Geometry: final body of the model. Coordinates: model frame, mm. A direction names the side the tool comes from. Round coordinates to 2 decimals unless told otherwise and drop trailing zeros. Loops run counter-clockwise (first coordinate to the right, second up) from the corner with the lowest first, then second, coordinate; pieces in that order, holes last. Notation, with made-up numbers: M 70,-7 L 124,-7 A19 cw 124,23 Z; hole C 89,15 d2. An arc over 180 degrees is marked long. Answer as a JSON object with one key per item and string values.
from build123d import *

# Parameters (mm, degrees)
F1_DEPTH = 96.75
F2_W     = 67
F2_H     = 15
F3_DEPTH = 2.5
F4_W     = 54
F4_H     = 1
F5_DEPTH = 88
F6_W     = 45
F6_H     = 77
F7_DEPTH = 1.5
F8_R     = 1
F9_R     = 2


with BuildPart() as f1:
    # F0 (on Front) → F1 (new body)
    with BuildSketch(Plane.XZ):
        Polygon((-27.75, 0), (-27.75, -3), (-30.75, -3), (-30.75, -4.5), (30.75, -4.5), (30.75, -3), (27.75, -3), (27.75, 0), align=None)
    extrude(amount=F1_DEPTH)

    # F2 (on face) → F3 (join)
    with BuildSketch(Plane.XZ.offset(96.75)):
        with Locations((0, -8.5)):
            Rectangle(F2_W, F2_H)
    extrude(amount=F3_DEPTH)

    # F4 (on face) → F5 (cut)
    with BuildSketch(Plane(origin=(0, 0, 0), x_dir=(-1, 0, 0), z_dir=(0, 1, 0))):
        with Locations((0, -2)):
            Rectangle(F4_W, F4_H)
    extrude(amount=-F5_DEPTH, mode=Mode.SUBTRACT)

    # F6 (on face) → F7 (cut, through all)
    with BuildSketch(Plane.XY):
        with Locations((0, -42.5)):
            Rectangle(F6_W, F6_H)
    extrude(amount=-F7_DEPTH, mode=Mode.SUBTRACT)

    # F8
    f8_edges = [f1.edges().sort_by_distance(p)[0] for p in [
        (-22.5, -81, -0.75),
        (-22.5, -4, -0.75),
        (22.5, -4, -0.75),
        (22.5, -81, -0.75),
    ]]
    fillet(f8_edges, radius=F8_R)

    # F9
    f9_edges = [f1.edges().sort_by_distance(p)[0] for p in [
        (0, -99.25, -16),
        (0, -99.25, -1),
        (33.5, -99.25, -8.5),
        (-33.5, -99.25, -8.5),
    ]]
    fillet(f9_edges, radius=F9_R)


solid = f1.part
1) Section query D-D (z = -8.5). Return the cut outline in (x, y).
Results:
{"outline": "M -33.5,-97.25 A2 ccw -31.5,-99.25 L 31.5,-99.25 A2 ccw 33.5,-97.25 L 33.5,-96.75 L -33.5,-96.75 Z"}
2) Section query C-C (x = 24). Return the cut outline in (y, z), and give its area (3 significant figures).
Results:
{"outline": "M -99.25,-14 A2 ccw -97.25,-16 L -96.75,-16 L -96.75,-4.5 L 0,-4.5 L 0,-2.5 L -88,-2.5 L -88,-1.5 L 0,-1.5 L 0,0 L -96.75,0 L -96.75,-1 L -97.25,-1 A2 ccw -99.25,-3 Z", "area": "383 mm2"}
3) Ray query, line 1 (Z direction, x = -24.5, y = -19.5); line 2 (X direction, y = -68, z = -1); line 3 (Y direction, x = 23, z = -8.75). Return the intervals inside material, ascending.
Results:
{"line 1": "-4.5 to -2.5, -1.5 to 0", "line 2": "-27.75 to -22.5, 22.5 to 27.75", "line 3": "-99.25 to -96.75"}
4) Pin query (flat end, axial travel): P1, Ø1.5, axis at y = -31.5, z = -1, coming from the -X side; P2, Ø1.2, axis at y = -64.5, z = -4, coming from the -X side; P3, Ø0.9, axis at x = 28.5, y = -64, coming from the +Z side. Return the tip coordinate at first contact, or that it passes through.
Results:
{"P1": "x = -27.75", "P2": "x = -30.75", "P3": "z = -3"}
5) Section query A-A (x = 1). Return the cut outline in (y, z), and give its area (3 significant figures).
Results:
{"outline": "M -99.25,-14 A2 ccw -97.25,-16 L -96.75,-16 L -96.75,-4.5 L 0,-4.5 L 0,-2.5 L -88,-2.5 L -88,-1.5 L -81,-1.5 L -81,0 L -96.75,0 L -96.75,-1 L -97.25,-1 A2 ccw -99.25,-3 Z; M -4,-1.5 L 0,-1.5 L 0,0 L -4,0 Z", "area": "268 mm2"}
6) Pull-direction query (X, two-part tool) for faces 1 (the flat face through (0, -43, -2.5)), 2 (the flat face through (-27.75, -48, -1)), 3 (the flat face through (0, -99.25, -8)); classes: +X half, -X half, draft (parallel to the pull), parting line (faces both ways), or undercut.
Results:
{"face 1": "undercut", "face 2": "-X half", "face 3": "draft"}
7) Section query B-B (y = -90). Return the cut outline in (x, z).
Results:
{"outline": "M -30.75,-4.5 L 30.75,-4.5 L 30.75,-3 L 27.75,-3 L 27.75,0 L -27.75,0 L -27.75,-3 L -30.75,-3 Z"}
8) Reachability of faces 4 (the flat face through (0, -48, -4.5)), 5 (the flat face through (24, -47, -1.5)), 6 (the flat face through (-29, -48, -3)), 7 (the flat face through (29, -48, -3)) from +Z, -Z, +X, -X, +Y, -Y: full face, straight path, thin tool, end or side. Return the list, or none.
Results:
{"face 4": "-Z, +X, -X, +Y", "face 5": "+Y", "face 6": "+Z, -X, +Y", "face 7": "+Z, +X, +Y"}
